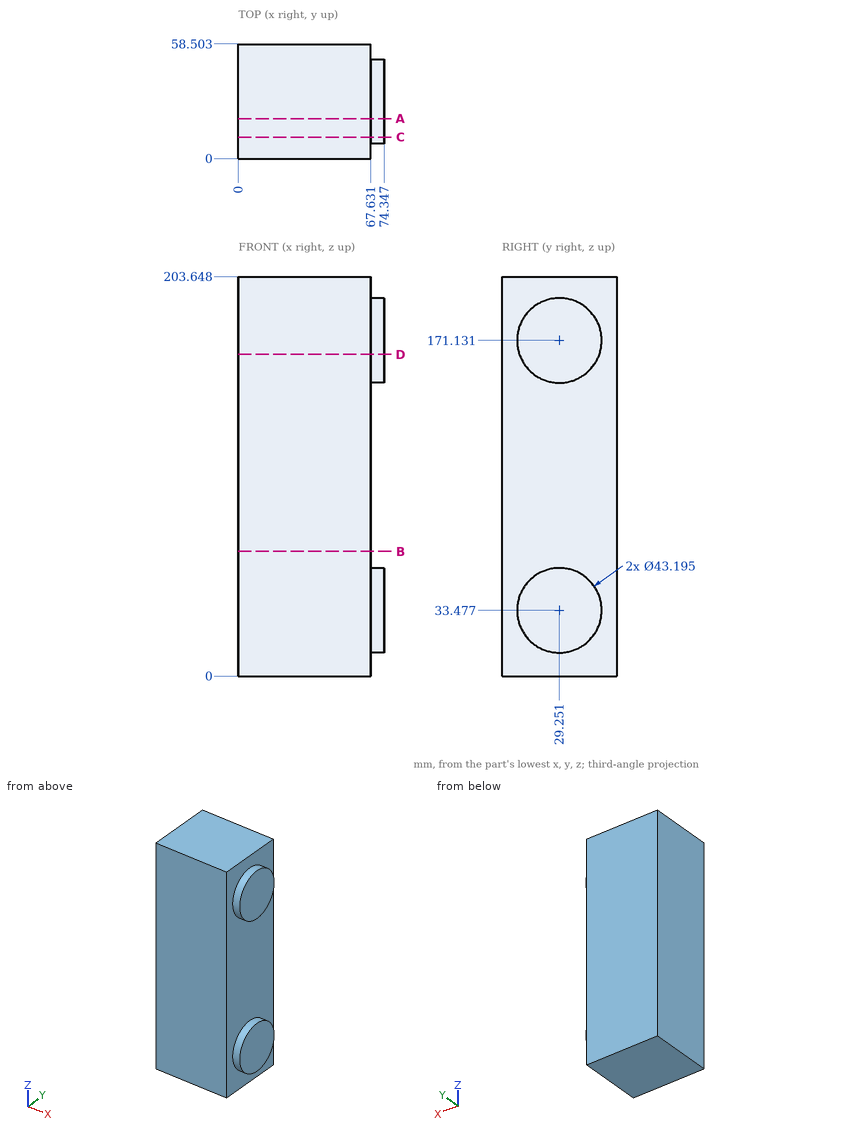
Geometry check sheet. Reference: drawing and pictorial views, mm from the part's lowest x, y, z. Give positions to 0.01 mm unless a question says otherwise; leave off trailing zeros. Order: outer loops, then holes, each group sorted by start corner. A loop starts at its lowest first (then second) coordinate and runs counter-clockwise, first axis right, second up. Notation, with made-up numbers: M 85.5,8 L 112.5,8 A14 cw 112.5,29 Z; hole C -17,23.25 d7. An arc over 180 degrees is marked long. Answer as a JSON object with one key per item and string values. Group by question number.
1) Cross-section at D-D (z = 164). Enter the section's corners in (x, y) (1 decimal).
2) Cross-section at A-A (y = 20.5). Enter the section's corners in (x, z) (1 decimal).
3) Cross-section at C-C (y = 11). Enter the section's corners in (x, z) (1 decimal), then the cut area to 3 significant figures.
4) Depth check by flat-ended pin: pin 1 Ø10 at (y, z) = (45.5, 64) entering from +X. Enter the tip coordinate at first touch or a pass-through.
5) Cross-section at B-B (z = 63.5). Enter the section's corners in (x, y).
6) Scan lines: line 1 along X through (y, z) = (16.5, 71); line 2 along Z through (x, y) = (69.5, 27). Record each from-to range of solid material in increasing order. Write a range as [from, to].
Result sheet:
{
 "1": {"outline": "M 0,0 L 67.6,0 L 67.6,8.9 L 74.3,8.9 L 74.3,49.6 L 67.6,49.6 L 67.6,58.5 L 0,58.5 Z"},
 "2": {"outline": "M 0,0 L 67.6,0 L 67.6,13.7 L 74.3,13.7 L 74.3,53.2 L 67.6,53.2 L 67.6,151.4 L 74.3,151.4 L 74.3,190.9 L 67.6,190.9 L 67.6,203.6 L 0,203.6 Z"},
 "3": {"outline": "M 0,0 L 67.6,0 L 67.6,21.9 L 74.3,21.9 L 74.3,45 L 67.6,45 L 67.6,159.6 L 74.3,159.6 L 74.3,182.7 L 67.6,182.7 L 67.6,203.6 L 0,203.6 Z", "area": "14,100 mm2"},
 "4": {"pin 1": "stops at x = 67.63"},
 "5": {"outline": "M 0,0 L 67.63,0 L 67.63,58.5 L 0,58.5 Z"},
 "6": {"line 1": "x = [0, 67.63]", "line 2": "z = [12, 54.96], [149.65, 192.61]"}
}
